```python
from build123d import *

# Parameters (mm, degrees)
SKETCH_1_W         = 30.5
SKETCH_1_H         = 8
EXTRUDE_1_DEPTH    = 8
HOLE_WIZARD_M4_1_D = 3.3
HOLE_WIZARD_M4_2_D = 3.3


with BuildPart() as part:
    # 草图1 → 凸台-拉伸1 (new body)
    with BuildSketch(Plane.XY):
        Rectangle(SKETCH_1_W, SKETCH_1_H)
    extrude(amount=EXTRUDE_1_DEPTH)

    # M4 螺纹孔1 (through all)
    with Locations(Plane(origin=(3.75, 0, 8), x_dir=(1, 0, 0), z_dir=(0, 0, 1))):
        with Locations((0, 0), (-15, 0)):
            Hole(HOLE_WIZARD_M4_1_D / 2)

    # M4 螺纹孔2 (through all)
    with Locations(Plane(origin=(-3.75, 4, 4), x_dir=(0, 0, 1), z_dir=(0, 1, 0))):
        with Locations((0, 0), (0, 15)):
            Hole(HOLE_WIZARD_M4_2_D / 2)


solid = part.part
```
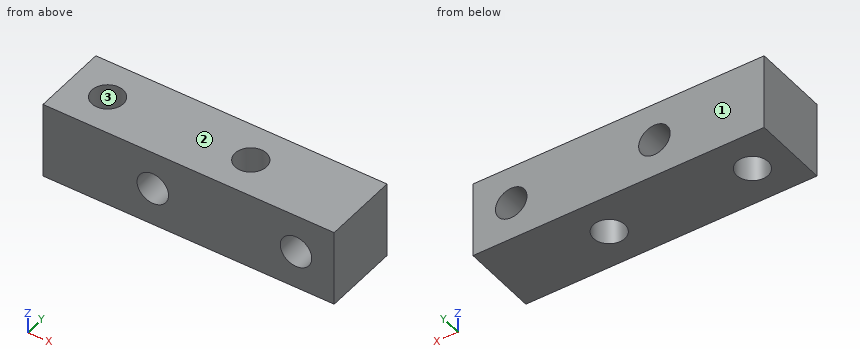
Build history of the part. All positions in model axes, mm. Face numbers are marked on the shaded views. Give positions to 0.01 mm unless a question says otherwise; leave off trailing zeros. Loops run counter-clockwise (first coordinate to the right, second up) from the corner with the lowest first, then second, coordinate; pieces in that order, holes last.
Item 1: Slice it at D-D, the plane z = 6.25. List the corners of the cut face in (x, y), and give its area (3 significant figures).
Answers follow:
outline: (-15.25, -4) - (15.25, -4) - (15.25, 4) - (-15.25, 4) - close; hole circle Ø3.3 at (-11.25, 0); hole circle Ø3.3 at (3.75, 0)
area: 227 mm2
Item 2: Slice it at B-B, the plane y = 0. List the corners of the cut face in (x, z).
Answers follow:
outline: (-15.25, 0) - (-12.9, 0) - (-12.9, 8) - (-15.25, 8) - close; (-9.6, 0) - (2.1, 0) - (2.1, 8) - (-9.6, 8) - close; (5.4, 0) - (15.25, 0) - (15.25, 8) - (5.4, 8) - close; hole circle Ø3.3 at (-3.75, 4); hole circle Ø3.3 at (11.25, 4)
Item 3: Slice it at A-A, the plane z = 4. List the corners of the cut face in (x, y).
Answers follow:
outline: (-15.25, -4) - (-5.4, -4) - (-5.4, 4) - (-15.25, 4) - close; (-2.1, -4) - (9.6, -4) - (9.6, 4) - (-2.1, 4) - close; (12.9, -4) - (15.25, -4) - (15.25, 4) - (12.9, 4) - close; hole circle Ø3.3 at (-11.25, 0); hole circle Ø3.3 at (3.75, 0)
Item 4: Drill centre lines: line 1 (X direction, y = -0.25, z = 3.5); line 2 (X direction, y = 2.5, z = 2.75); line 3 (Y direction, x = 3.75, z = 6.25). Where is each one in solid material? Low to high.
Answers follow:
line 1: x = -15.25 to -12.88, -9.62 to -5.32, -2.18 to 2.12, 5.38 to 9.68, 12.82 to 15.25
line 2: x = -15.25 to -4.83, -2.67 to 10.17, 12.33 to 15.25
line 3: y = -4 to -1.65, 1.65 to 4
Item 5: Slice it at C-C, the plane x = -3.75. List the corners of the cut face in (y, z), and give its area (3 significant figures).
Answers follow:
outline: (-4, 0) - (4, 0) - (4, 2.35) - (-4, 2.35) - close; (-4, 5.65) - (4, 5.65) - (4, 8) - (-4, 8) - close
area: 37.6 mm2
Item 6: Pull direction Y, two halves, no side cores. Call the marked faces 1, 2 and 3: released by +Y, released by -Y, zero draft, split by the parting line, or undercut.
Answers follow:
face 1: released by +Y
face 2: zero draft
face 3: undercut
